Can you work these out from the drawing? Everything is in mm from the part's minimum corner. Round coordinates to 2 decimals unless told otherwise and drop trailing zeros. Loops run counter-clockwise (first coordinate to the right, second up) from the corner with the lowest first, then second, coordinate; pieces in that order, holes last. Notation, with made-up numbers: M 37,69.5 L 84,69.5 A11 cw 84,82.5 Z; hole C 38,-31 d6. An arc over 180 degrees is marked long. Use a Markdown table: item, result.
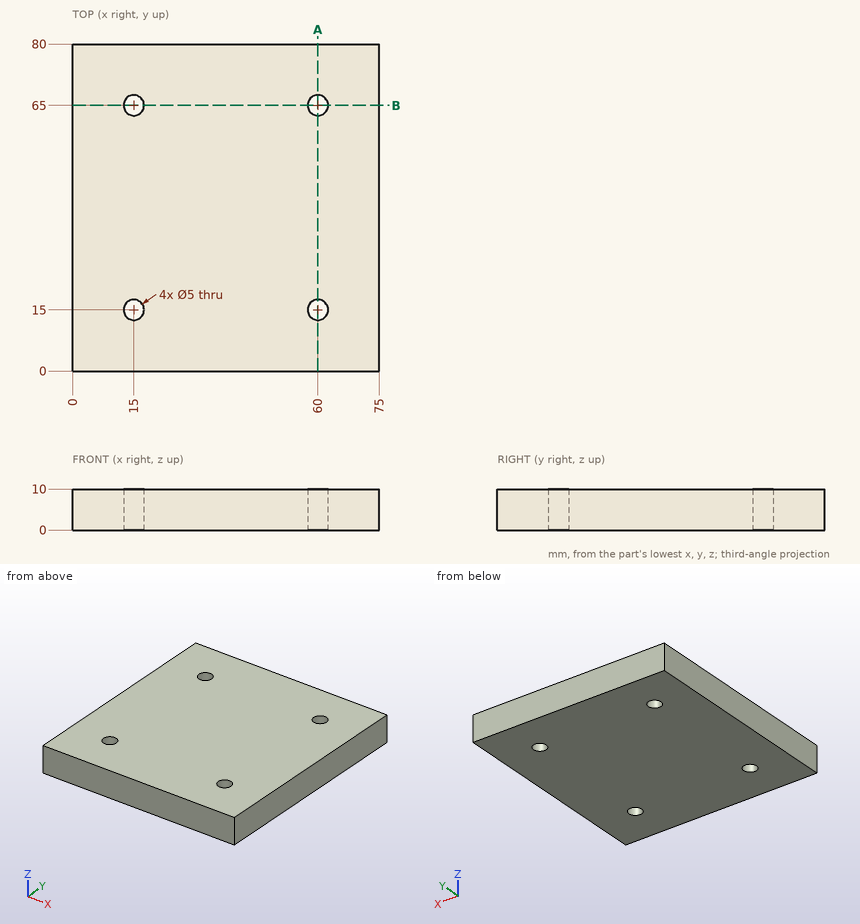
Q1. Imagine slicing it at B-B, the plane y = 65. Please give me the cut outline in (x, z).
Return value:
| item | result |
|---|---|
| outline | M 0,0 L 12.5,0 L 12.5,10 L 0,10 Z; M 17.5,0 L 57.5,0 L 57.5,10 L 17.5,10 Z; M 62.5,0 L 75,0 L 75,10 L 62.5,10 Z |
Q2. Imagine slicing it at A-A, the plane x = 60. Please give me the cut outline in (y, z), then the cut area to 3 significant figures.
Return value:
| item | result |
|---|---|
| outline | M 0,0 L 12.5,0 L 12.5,10 L 0,10 Z; M 17.5,0 L 62.5,0 L 62.5,10 L 17.5,10 Z; M 67.5,0 L 80,0 L 80,10 L 67.5,10 Z |
| area | 700 mm^2 |
Q3. Will this pin go through, and if not, where does the flat tip stop? P1, Ø4.5, axis at x = 15, y = 65, coming from the +Z side.
Return value:
| item | result |
|---|---|
| P1 | passes through |
Q4. I need wall thicknesses on line 1 (Y direction, x = 60, z = 7); line 2 (Y direction, x = 14, z = 7.5). Which ranges of each line are inside material? Lowest first, please. Write a range as from..to.
Return value:
| item | result |
|---|---|
| line 1 | y = 0..12.5, 17.5..62.5, 67.5..80 |
| line 2 | y = 0..12.71, 17.29..62.71, 67.29..80 |
